The model under review builds one solid part; all positions refer to its coordinate system, in mm. Coordinates: 2 decimals unless noted, no trailing zeros. Write each loop counter-clockwise with the first axis right and the second up, starting at its lowest first coordinate (ties: lowest second). Pieces come first, ordered by that corner, then holes.
1) For line 1 (Y direction, x = 2, z = -2); line 2 (Y direction, x = 3.75, z = -19.5); line 3 (Z direction, x = 2.85, y = 83), list the stretches that pass through material, from the lowest coordinate up.
2) Add section D-D, the plane y = 61.5. State the section outline as (x, z) points.
3) Add section C-C, the plane z = 77. State the section outline as (x, y) points.
4) Add section A-A, the plane y = -75.5. State the section outline as (x, z) points, then the cut area to 3 significant figures.
5) For P1, Ø3.5, axis at y = -92.08, z = -14.8, coming from the -X side, flat-tipped, find the tip position at first contact; note if it passes through.
6) Add section B-B, the plane x = 3.4. Give the number of separate pieces and of enclosed holes in the cut face, then the cut area to 3 significant figures.
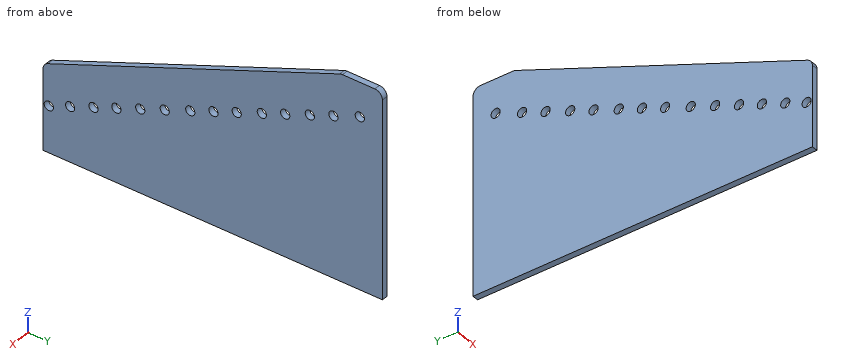
from build123d import *

# Parameters (mm, degrees)
F0_R     = 3.100498
F1_DEPTH = 4.064
F2_R     = 5.08


with BuildPart() as f1:
    # F0 (on Right) → F1 (new body)
    with BuildSketch(Plane.YZ):
        Polygon((-110.349961, 5.712933), (-110.349961, -51.461264), (118.143998, -51.461264), (118.143998, 85.298181), (90.28247, 85.298181), align=None)
        with Locations((-106.447847, -20.505097)):
            Circle(F0_R, mode=Mode.SUBTRACT)
        with Locations((-92.076812, -14.804511)):
            Circle(F0_R, mode=Mode.SUBTRACT)
        with Locations((-76.339489, -8.561957)):
            Circle(F0_R, mode=Mode.SUBTRACT)
        with Locations((-60.95832, -2.46068)):
            Circle(F0_R, mode=Mode.SUBTRACT)
        with Locations((-44.866651, 3.922433)):
            Circle(F0_R, mode=Mode.SUBTRACT)
        with Locations((-28.430619, 10.442145)):
            Circle(F0_R, mode=Mode.SUBTRACT)
        with Locations((-11.20806, 17.27385)):
            Circle(F0_R, mode=Mode.SUBTRACT)
        with Locations((4.416042, 23.471493)):
            Circle(F0_R, mode=Mode.SUBTRACT)
        with Locations((20.038726, 29.668572)):
            Circle(F0_R, mode=Mode.SUBTRACT)
        with Locations((36.965934, 36.38312)):
            Circle(F0_R, mode=Mode.SUBTRACT)
        with Locations((52.71062, 42.628594)):
            Circle(F0_R, mode=Mode.SUBTRACT)
        with Locations((69.271646, 49.197888)):
            Circle(F0_R, mode=Mode.SUBTRACT)
        with Locations((85.138393, 55.491781)):
            Circle(F0_R, mode=Mode.SUBTRACT)
        with Locations((102.904496, 62.539094)):
            Circle(F0_R, mode=Mode.SUBTRACT)
    extrude(amount=F1_DEPTH)

    # F2
    f2_edges = [f1.edges().sort_by_distance(p)[0] for p in [
        (2.032, -110.349961, 5.712933),
        (2.032, 118.143998, 85.298181),
        (2.032, 90.28247, 85.298181),
    ]]
    fillet(f2_edges, radius=F2_R)


solid = f1.part
Geometry results:
1. line 1: y = -110.35 to -64.02, -57.89 to 118.14
1. line 2: y = -110.35 to -109.38, -103.51 to 118.14
1. line 3: z = -51.46 to 53.25, 57.74 to 82.41
2. outline: (0, -51.46) - (4.06, -51.46) - (4.06, 73.88) - (0, 73.88) - close
3. outline: (0, 69.36) - (4.06, 69.36) - (4.06, 118.14) - (0, 118.14) - close
4. outline: (0, -51.46) - (4.06, -51.46) - (4.06, -11.55) - (0, -11.55) - close; (0, -5.58) - (4.06, -5.58) - (4.06, 19.54) - (0, 19.54) - close
4. area: 264 mm2
5. P1: passes through
6. separate pieces: 1
6. enclosed holes: 14
6. area: 22,800 mm2
